Source: CAD feature listing. Evaluate the final solid. Frame: model axes, mm. Face numbers are marked on the shaded views. Give positions to 0.01 mm unless a question says otherwise; leave off trailing zeros. Loops run counter-clockwise (first coordinate to the right, second up) from the corner with the lowest first, then second, coordinate; pieces in that order, holes last.
from build123d import *


with BuildPart() as part:
    # Sketch1 → Revolve1 (revolve)
    with BuildSketch(Plane.XY):
        with BuildLine():
            Line((-19.513838733, 23.330040777), (-19.513838733, 26.330040777))
            Line((-19.513838733, 26.330040777), (-21.513838733, 26.330040777))
            Line((-21.513838733, 26.330040777), (-27.138378423, 23.330040777))
            Line((-27.138378423, 23.330040777), (-29.513838733, 21.835217327))
            Line((-29.513838733, 21.835217327), (-29.513838733, -18.669959223))
            Line((-29.513838733, -18.669959223), (12.986161267, -18.669959223))
            Line((12.986161267, -18.669959223), (12.986161267, -12.147726016))
            ThreePointArc((12.986161267, -12.147726016), (-5.743453451, -2.097812317), (-7.724873095, 19.065202805))
            Line((-7.724873095, 19.065202805), (-8.991099708, 20.330040777))
            Line((-8.991099708, 20.330040777), (-19.498450474, 20.330040777))
            Line((-19.498450474, 20.330040777), (-19.513838733, 23.330040777))
        make_face()
    revolve(axis=Axis((12.986161267, -12.147726016, 0), (0, -1, 0)))


solid = part.part
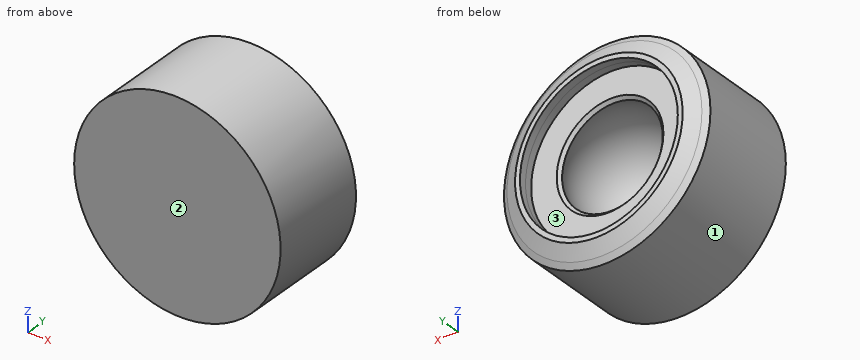
1) Pull-direction query (X, two-part tool) for the marked faces 1, 2 and 3; classes: released by +X, released by -X, zero draft, split by the parting line, or undercut.
Checks:
face 1: split by the parting line
face 2: zero draft
face 3: undercut
2) Ray query, probe 1 along Y at (x, z) = (31.5, 13); probe 2 along X at (y, z) = (24.4, 0); probe 3 along Z at (x, y) = (20, 11.5). Return the intervals inside material, ascending.
Checks:
probe 1: y = -18.67 to 20.33
probe 2: x = -25.13 to -19.51, 45.49 to 51.1
probe 3: z = -41.92 to -21.32, 21.32 to 41.92
3) Contact query for flat-ended pins moving along their axis: P1, Ø10, axis at x = 44, z = -25, coming from the +Y side; P2, Ø1.5, axis at x = 28.5, y = -4.5, coming from the +Z side; P3, Ø1.5, axis at y = -13, z = -10.5, coming from the +X side. Output: stop coordinate, or through.
Checks:
P1: stops at y = 26.15
P2: stops at z = 39.85
P3: stops at x = 54.35
4) Cut plane A-A (y = -6.5). Return loops of the section in (x, z), and give its area (3 significant figures).
Checks:
outline: circle Ø85 at (12.99, 0); hole circle Ø29.8 at (12.99, 0)
area: 4,980 mm2
